from build123d import *

# Parameters (mm, degrees)
SKETCH_1_W         = 24
SKETCH_1_H         = 24
SKETCH_1_W_2       = 20
SKETCH_1_H_2       = 20
EXTRUDE_1_DEPTH    = 45.005
HOLE_WIZARD_M3_1_D = 2.5
HOLE_WIZARD_M3_2_D = 2.5


with BuildPart() as part:
    # 草图1 → 凸台-拉伸1 (new, symmetric)
    with BuildSketch(Plane.XY):
        Rectangle(SKETCH_1_W, SKETCH_1_H)
        Rectangle(SKETCH_1_W_2, SKETCH_1_H_2, mode=Mode.SUBTRACT)
    extrude(amount=EXTRUDE_1_DEPTH, both=True)

    # M3 螺纹孔的螺纹孔钻头1 (through all)
    with Locations(Plane(origin=(-12, 0, -33.005), x_dir=(0, -1, 0), z_dir=(-1, 0, 0))):
        with Locations((0, 0)):
            hole_wizard_m3_1 = Hole(HOLE_WIZARD_M3_1_D / 2)

    # 镜向1: M3 螺纹孔的螺纹孔钻头1 across plane
    add(hole_wizard_m3_1.mirror(Plane.XY), mode=Mode.SUBTRACT)

    # M3 螺纹孔的螺纹孔钻头2 (through all)
    with Locations(Plane(origin=(0, 12, -33.005), x_dir=(0, 0, 1), z_dir=(0, 1, 0))):
        with Locations((0, 0)):
            hole_wizard_m3_2 = Hole(HOLE_WIZARD_M3_2_D / 2)

    # 镜向2: M3 螺纹孔的螺纹孔钻头2 across plane
    add(hole_wizard_m3_2.mirror(Plane.XY), mode=Mode.SUBTRACT)


solid = part.part
Verification items for the finished model (mm, model axes). A direction names the side the tool comes from. Give positions to 0.01 mm unless a question says otherwise; leave off trailing zeros. Loops run counter-clockwise (first coordinate to the right, second up) from the corner with the lowest first, then second, coordinate; pieces in that order, holes last. Notation, with made-up numbers: (86.5, 53.25) - (130.5, 53.25) arc R11 cw to (130.5, 64.25) - close; hole circle Ø5 at (28, 32.5). An arc over 180 degrees is marked (long way). Write each question's results on one line, items separated by ' | '.
1) Sectioned sample at C-C on z = -20. Record the boundary of the cut face in (x, y), plus the area to 3 significant figures.
Solution:
outline: (-12, -12) - (12, -12) - (12, 12) - (-12, 12) - close; hole (-10, -10) - (10, -10) - (10, 10) - (-10, 10) - close | area: 176 mm2
2) Tool access check on faces 1 (the flat face through (0, -10, 1)), 2 (the cylindrical face through (-10.986, -0.271, -34.225)). Record the directions out of +Z, -Z, +X, -X, +Y, -Y that give a thin tool (end or side, any length) a straight path to the whole face; none if there is none.
Solution:
face 1: +Z, -Z | face 2: +X, -X
3) Sectioned sample at B-B on y = 0. Record the boundary of the cut face in (x, z) (3 decimals), plus the area to 3 significant figures.
Solution:
outline: (-12, -45.005) - (-10, -45.005) - (-10, -34.255) - (-12, -34.255) - close; (-12, -31.755) - (-10, -31.755) - (-10, 31.755) - (-12, 31.755) - close; (-12, 34.255) - (-10, 34.255) - (-10, 45.005) - (-12, 45.005) - close; (10, -45.005) - (12, -45.005) - (12, -34.255) - (10, -34.255) - close; (10, -31.755) - (12, -31.755) - (12, 31.755) - (10, 31.755) - close; (10, 34.255) - (12, 34.255) - (12, 45.005) - (10, 45.005) - close | area: 340 mm2
4) Material ranges on L1, parallel to Z at x = -11.05, y = 0 (3 decimals); L2, parallel to Y at x = -6, z = 27, recorded low to high. Write a range as from..to.
Solution:
L1: -45.005..-34.255, -31.755..31.755, 34.255..45.005 | L2: -12..-10, 10..12
5) Mould release check, pull along X, two halves, no side actions. Record for faces 3 (the cylindrical face through (0.375, -11.014, -34.197)), 4 (the cylindrical face through (-0.48, -11.01, 34.16)), 5 (the flat face through (-12, 0, 1)), 6 (the flat face through (10.5, 0.2, 45.005)): pulls with the +X half, pulls with the -X half, needs draft (parallel to the pull), parting line crosses it, or undercut.
Solution:
face 3: undercut | face 4: undercut | face 5: pulls with the -X half | face 6: needs draft
6) Sectioned sample at A-A on x = 7.25. Record the boundary of the cut face in (y, z) (3 decimals).
Solution:
outline: (-12, -45.005) - (-10, -45.005) - (-10, 45.005) - (-12, 45.005) - close; (10, -45.005) - (12, -45.005) - (12, 45.005) - (10, 45.005) - close
